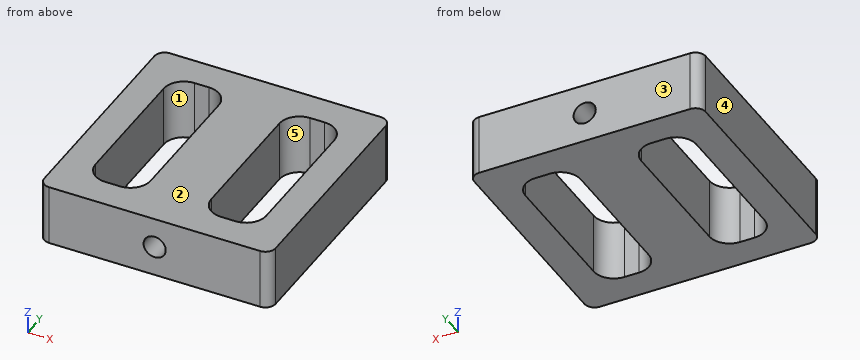
```python
from build123d import *

# Parameters (mm, degrees)
SKETCH_1_W          = 22.9
SKETCH_1_H          = 22.9
EXTRUDE_1_DEPTH     = 6
SKETCH_2_R          = 1.1
CUT_EXTRUDE_1_DEPTH = 27.296625259
SKETCH_3_W          = 5.45
SKETCH_3_H          = 16.9
CUT_EXTRUDE_2_DEPTH = 6
FILLET_1_R          = 2
FILLET_2_R          = 1


with BuildPart() as part:
    # 草图1 → 凸台-拉伸1 (new body)
    with BuildSketch(Plane.XY):
        Rectangle(SKETCH_1_W, SKETCH_1_H)
    extrude(amount=EXTRUDE_1_DEPTH)

    # 草图2 → 切除-拉伸1 (cut, through all)
    with BuildSketch(Plane(origin=(0, 11.45, 0), x_dir=(1, 0, 0), z_dir=(0, 1, 0))):
        with Locations(Location((0, -3, 0), (0, 0, 180))):
            Circle(SKETCH_2_R)
    extrude(amount=-CUT_EXTRUDE_1_DEPTH, mode=Mode.SUBTRACT)

    # 草图3 → 切除-拉伸2 (cut)
    with BuildSketch(Plane(origin=(0, 0, 0), x_dir=(-1, 0, 0), z_dir=(0, 0, -1))):
        with Locations((5.725, 0)):
            Rectangle(SKETCH_3_W, SKETCH_3_H)
        with Locations((-5.725, 0)):
            Rectangle(SKETCH_3_W, SKETCH_3_H)
    extrude(amount=-CUT_EXTRUDE_2_DEPTH, mode=Mode.SUBTRACT)

    # 圆角1
    fillet_1_edges = [part.edges().sort_by_distance(p)[0] for p in [
        (-8.45, 8.45, 3),
        (-8.45, -8.45, 3),
        (-3, -8.45, 3),
        (-3, 8.45, 3),
        (3, 8.45, 3),
        (3, -8.45, 3),
        (8.45, -8.45, 3),
        (8.45, 8.45, 3),
    ]]
    fillet(fillet_1_edges, radius=FILLET_1_R)

    # 圆角2
    fillet_2_edges = [part.edges().sort_by_distance(p)[0] for p in [
        (-11.45, 11.45, 3),
        (11.45, 11.45, 3),
        (11.45, -11.45, 3),
        (-11.45, -11.45, 3),
    ]]
    fillet(fillet_2_edges, radius=FILLET_2_R)


solid = part.part
```
CAD build for the part. Positions are in the model's coordinates, mm. Face numbers are marked on the shaded views. A direction names the side the tool comes from. Coordinates: 2 decimals unless noted, no trailing zeros. Write each loop counter-clockwise with the first axis right and the second up, starting at its lowest first coordinate (ties: lowest second). Pieces come first, ordered by that corner, then holes.
(1) Cut at B-B, the plane x = 0. List the corners of the cut face in (y, z), and give its area (3 significant figures).
(2) Drill centre lines: probe 1 along X at (y, z) = (-1.5, 1.45); probe 2 along Z at (x, y) = (0, -3); probe 3 along Y at (x, z) = (-6.5, 5.7). Where is each one in solid material? Low to high.
(3) Flat gauge pin, fed straight in: pin 1 (5 mm diameter, centred on x = 0, y = -7.5, fed in from -Z). Where does the tip first touch, or does it go through?
(4) Cut at C-C, the plane y = 5.5. List the corners of the cut face in (x, z).
(5) Two-plate mould, pull along Y, no slides. Class the marked faces 3, 4 and 5: +Y half, -Y half, draft (parallel to the pull), parting line (faces both ways), or undercut.
(6) Cut at A-A, the plane z = 3. List the corners of the cut face in (x, y).
(7) Cut at D-D, the plane z = 1.1. List the corners of the cut face in (x, y).
(8) 3-axis set-ups, long thin cutter, end or side, ignore diameter. For the marked faces 1 and 2: which of +Z, -Z, +X, -X, +Y, -Y reach the whole face in a straight line?
Geometry says:
1. outline: (-11.45, 0) - (11.45, 0) - (11.45, 1.9) - (-11.45, 1.9) - close; (-11.45, 4.1) - (11.45, 4.1) - (11.45, 6) - (-11.45, 6) - close
1. area: 87.0 mm2
2. probe 1: x = -11.45 to -8.45, -3 to 3, 8.45 to 11.45
2. probe 2: z = 0 to 1.9, 4.1 to 6
2. probe 3: y = -11.45 to -8.45, 8.45 to 11.45
3. pin 1: stops at z = 0
4. outline: (-11.45, 0) - (-8.45, 0) - (-8.45, 6) - (-11.45, 6) - close; (-3, 0) - (3, 0) - (3, 6) - (-3, 6) - close; (8.45, 0) - (11.45, 0) - (11.45, 6) - (8.45, 6) - close; hole circle Ø2.2 at (0, 3)
5. face 3: +Y half
5. face 4: draft
5. face 5: undercut
6. outline: (-11.45, -10.45) arc R1 ccw to (-10.45, -11.45) - (-1.1, -11.45) - (-1.1, 11.45) - (-10.45, 11.45) arc R1 ccw to (-11.45, 10.45) - close; (1.1, -11.45) - (10.45, -11.45) arc R1 ccw to (11.45, -10.45) - (11.45, 10.45) arc R1 ccw to (10.45, 11.45) - (1.1, 11.45) - close; hole (-8.45, -6.45) arc R2 ccw to (-6.45, -8.45) - (-5, -8.45) arc R2 ccw to (-3, -6.45) - (-3, 6.45) arc R2 ccw to (-5, 8.45) - (-6.45, 8.45) arc R2 ccw to (-8.45, 6.45) - close; hole (3, -6.45) arc R2 ccw to (5, -8.45) - (6.45, -8.45) arc R2 ccw to (8.45, -6.45) - (8.45, 6.45) arc R2 ccw to (6.45, 8.45) - (5, 8.45) arc R2 ccw to (3, 6.45) - close
7. outline: (-11.45, -10.45) arc R1 ccw to (-10.45, -11.45) - (10.45, -11.45) arc R1 ccw to (11.45, -10.45) - (11.45, 10.45) arc R1 ccw to (10.45, 11.45) - (-10.45, 11.45) arc R1 ccw to (-11.45, 10.45) - close; hole (-8.45, -6.45) arc R2 ccw to (-6.45, -8.45) - (-5, -8.45) arc R2 ccw to (-3, -6.45) - (-3, 6.45) arc R2 ccw to (-5, 8.45) - (-6.45, 8.45) arc R2 ccw to (-8.45, 6.45) - close; hole (3, -6.45) arc R2 ccw to (5, -8.45) - (6.45, -8.45) arc R2 ccw to (8.45, -6.45) - (8.45, 6.45) arc R2 ccw to (6.45, 8.45) - (5, 8.45) arc R2 ccw to (3, 6.45) - close
8. face 1: +Z, -Z
8. face 2: +Z, +X, -X, +Y, -Y
